Solid Edge part; units mm, degrees
sketch "Sketch1" plane through (0, 0, 0) normal (0, -1, 0) x (1, 0, 0)
  line L0 (0, 30) -> (0, 20)
  line L1 (0, -20) -> (0, -30)
  arc A0 (0, -20) -> (0, 20) centre (0, 0) cw
  arc A1 (0, -30) -> (0, 30) centre (0, 0) cw
revolve "RevolvedProtrusion1" add sketch "Sketch1" angle 360 about axis through (0, 0, 30) along (0, 0, -1)
sketch "Sketch2" plane through (0, 0, 0) normal (0, 0, 1) x (1, 0, 0)
  circle A0 centre (0, 0) radius 5
extrude "Cutout1" cut sketch "Sketch2" along normal mid plane 93.4764
sketch "Sketch3" plane through (0, 0, 0) normal (0, -1, 0) x (1, 0, 0)
  circle A0 centre (0, 0) radius 5
extrude "ExtrudedCutout_2" cut sketch "Sketch3" along normal blind 58.5589
pattern_circular "Pattern1" count 8 over 360 about axis through (0, 0, 0) along (0, 0, -1) of "ExtrudedCutout_2"
sketch "Sketch4" plane through (0, 0, 0) normal (0.7071, 0, -0.7071) x (-0.7071, 0, -0.7071)
  circle A0 centre (0, 0) radius 5
extrude "ExtrudedCutout_3" cut sketch "Sketch4" against normal blind 59.1564
sketch "Sketch5" plane through (0, 0, 0) normal (0.7071, 0, -0.7071) x (-0.7071, 0, -0.7071)
  circle A0 centre (0, 0) radius 5
extrude "ExtrudedCutout_4" cut sketch "Sketch5" along normal blind 73.7345
pattern_circular "Pattern3" count 6 over 360 about axis through (0, 0, 21.2132) along (0, 0, -1) of "ExtrudedCutout_3"
pattern_circular "Pattern5" count 6 over 360 about axis through (0, 0, -20.9165) along (0, 0, -1) of "ExtrudedCutout_4"
Source: CAD feature listing. Evaluate the final solid. Frame: model axes, mm. Round coordinates to 2 decimals unless told otherwise and drop trailing zeros. Loops run counter-clockwise (first coordinate to the right, second up) from the corner with the lowest first, then second, coordinate; pieces in that order, holes last. Notation, with made-up numbers: M 19,77.5 L 32,77.5 A19 cw 32,106.5 Z; hole C 0,19 d3. An arc over 180 degrees is marked long. Return JSON: item names as keys, results as strings. Group by question number.
1. Section query A-A on x = 0. Output: boundary loops of the cut face in (y, z).
2. Mould query, pull axis X, two halves, no side actions, for faces 1 (the face through (-24.4, 1.08, 4.88)), 2 (the face through (-13.99, -20.52, 1.92)). Classes: released by +X, released by -X, zero draft, split by the parting line, or undercut.
3. Material intervals for line 1 along Y through (x, z) = (-4, -12); line 2 along Z through (x, y) = (-2.5, 11); line 3 along Y through (x, z) = (0, 26), sorted ascending. Write a range as from..to.
4. Section query B-B on y = 0. State how many separate pieces and enclosed holes the cut face has, and give its area (3 significant figures).
5. Pin query (flat end, axial travel): pin 1 (5 mm diameter, centred on x = -22, y = -8.5, fed in from +Z); pin 2 (1 mm diameter, centred on x = -20.5, y = -0.5, fed in from -Z); pin 3 (5 mm diameter, centred on y = -15, z = 21.5, fed in from -X). Return the tip coordinate at first contact, or that it passes through.
6. Section query C-C on z = -6. Output: boundary loops of the cut face in (x, y), and give its area (3 significant figures).
Checks:
{
 "1": {"outline": "M -29.58,-5 A30 ccw -5,-29.58 L -5,-19.36 A20 cw -19.36,-5 Z; M -29.58,5 L -19.36,5 A20 cw -5,19.36 L -5,29.58 A30 ccw Z; M 5,-29.58 A30 ccw 29.58,-5 L 19.36,-5 A20 cw 5,-19.36 Z; M 5,19.36 A20 cw 19.36,5 L 29.58,5 A30 ccw 5,29.58 Z"},
 "2": {"face 1": "zero draft", "face 2": "undercut"},
 "3": {"line 1": "y = -27.2..-15.61, 15.61..27.2", "line 2": "z = -27.8..-16.52, 16.52..27.8", "line 3": "y = -14.97..-5, 5..14.97"},
 "4": {"separate pieces": "8", "enclosed holes": "0", "area": "765 mm²"},
 "5": {"pin 1": "stops at z = 21.34", "pin 2": "stops at z = -13.97", "pin 3": "stops at x = -18.37"},
 "6": {"outline": "C 0,0 d58.79; hole C 0,0 d38.16", "area": "1,570 mm²"}
}
